Geometry: final body of the model. Coordinates: model frame, mm. Face numbers are marked on the shaded views. A direction names the side the tool comes from. Coordinates: 2 decimals unless noted, no trailing zeros. Loops run counter-clockwise (first coordinate to the right, second up) from the corner with the lowest first, then second, coordinate; pieces in that order, holes last. Notation, with made-up numbers: (-37.5, 69.5) -> (15.5, 69.5) arc R21 cw to (15.5, 77.5) -> close; hole circle Ø9 at (57.5, -8.75). An arc over 180 degrees is marked (long way). One line per item, written item: value. Start each with the question number.
Item 1: Set-up query: the marked faces 1 and 2. Return all of +Z, -Z, +X, -X, +Y, -Y with unobstructed straight access to the full face (end or side cutting, diameter ignored); none if empty.
Item 2: Section query B-B on z = 53. Return loops of the section in (x, y), then the cut area to 3 significant figures.
Item 3: Ray query, probe 1 along Z at (x, y) = (13, -5); probe 2 along Y at (x, z) = (7, 29); probe 3 along Y at (x, z) = (-4, 45.5). Return the intervals inside material, ascending. Write a range as from..to.
Item 4: Section query A-A on z = 24. Return loops of the section in (x, y), then the cut area to 3 significant figures.
Item 5: Mould query, pull axis X, two halves, no side actions, for the marked faces 3, 4 and 5. Classes: +X half, -X half, draft (parallel to the pull), parting line (faces both ways), or undercut.
Item 6: Contact query for flat-ended pins moving along their axis: pin 1 Ø1.5 at (x, y) = (-2, -15) entering from +Z; pin 2 Ø6 at (y, z) = (11, 25) entering from +X; pin 3 Ø8 at (x, z) = (-12, 13) entering from -Y; pin 4 Ø4 at (x, z) = (-14, 29.5) entering from +Y. Output: stop coordinate, or through.
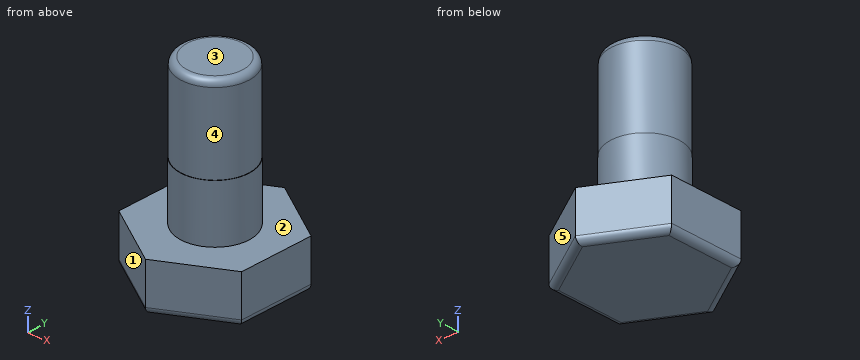
from build123d import *

# Parameters (mm, degrees)
EXTRUDE_430_DEPTH = 15
SKETCH_2_R        = 11
EXTRUDE_1_DEPTH   = 18
FILLET_3_R        = 2
SKETCH_3_R        = 10.9
EXTRUDE_1_2_DEPTH = 27
FILLET_4_R        = 2


with BuildPart() as part:
    # 草图1 → Extrude 430 (new body)
    with BuildSketch(Plane.XY):
        Polygon((20.472392036, 10.687118304), (0.980880074, 23.073170732), (-19.491511963, 12.386052428), (-20.472392036, -10.687118304), (-0.980880074, -23.073170732), (19.491511963, -12.386052428), align=None)
    extrude(amount=EXTRUDE_430_DEPTH)

    # 草图2 → Extrude 1 (add)
    with BuildSketch(Plane.XY.offset(15)):
        Circle(SKETCH_2_R)
    extrude(amount=EXTRUDE_1_DEPTH)

    # 圆角3
    fillet_3_edges = [part.edges().sort_by_distance(p)[0] for p in [
        (9.255315945, -17.72961158, 0),
        (-10.726636055, -16.880144518, 0),
        (-19.981952, 0.849467062, 0),
        (-9.255315945, 17.72961158, 0),
        (10.726636055, 16.880144518, 0),
        (19.981952, -0.849467062, 0),
    ]]
    fillet(fillet_3_edges, radius=FILLET_3_R)

    # 草图3 → Extrude 1 2 (add)
    with BuildSketch(Plane.XY.offset(33)):
        Circle(SKETCH_3_R)
    extrude(amount=EXTRUDE_1_2_DEPTH)

    # 圆角4
    fillet_4_edges = [part.edges().sort_by_distance(p)[0] for p in [
        (-10.9, 0, 60),
    ]]
    fillet(fillet_4_edges, radius=FILLET_4_R)


solid = part.part
Reply:
1. face 1: +Z, -Z, -X, -Y
1. face 2: +Z
2. outline: circle Ø21.8 at (0, 0)
2. area: 373 mm²
3. probe 1: z = 0..15
3. probe 2: y = -8.49..8.49
3. probe 3: y = -10.14..10.14
4. outline: circle Ø22 at (0, 0)
4. area: 380 mm²
5. face 3: draft
5. face 4: parting line
5. face 5: +X half
6. pin 1: stops at z = 15
6. pin 2: stops at x = 7.55
6. pin 3: stops at y = -18.61
6. pin 4: passes through
